Geometry: final body of the model. Coordinates: model frame, mm. Face numbers are marked on the shaded views. A direction names the side the tool comes from. Give positions to 0.01 mm unless a question says otherwise; leave off trailing zeros. Write each loop counter-clockwise with the first axis right and the second up, starting at its lowest first coordinate (ties: lowest second). Pieces come first, ordered by that corner, then holes. Notation, with made-up numbers: (68, 16) -> (98, 16) arc R21 ccw to (98, 55) -> close; hole circle Ø3 at (68, 38). An arc over 180 degrees is marked (long way). Answer as a JSON object with one key per item and string values. Group by question number.
(1) Contact query for flat-ended pins moving along their axis: pin 1 Ø2 at (x, y) = (2.5, 10) entering from +Z (3 decimals); pin 2 Ø10 at (x, z) = (4.5, 19.5) entering from +Y (3 decimals); pin 3 Ø2.5 at (x, y) = (0, 12.7) entering from +Z (1 decimal). Output: stop coordinate, or through.
(2) Set-up query: the marked faces 4 and 5. Return all of +Z, -Z, +X, -X, +Y, -Y with unobstructed straight access to the full face (end or side cutting, diameter ignored); none if empty.
(3) Draft query along Z for the marked faces 1, 2 and 3. Return one class per face: +Z half, -Z half, draft (parallel to the pull), parting line (faces both ways), or undercut.
(4) Section query A-A on y = 12.7. Output: boundary loops of the cut face in (x, z) (3 decimals).
(5) Section query B-B on z = -12.7. Output: boundary loops of the cut face in (x, y) (3 decimals), plus the area to 3 significant figures.
(6) Material intervals for probe 1 along Y at (x, z) = (0, -24.35); probe 2 along X at (y, z) = (12.7, -23.3); probe 3 along Y at (x, z) = (0, -23.5), sorted ascending.
(7) Section query C-C on x = -9. Output: boundary loops of the cut face in (y, z) (3 decimals).
(8) Section query D-D on y = 28. Output: boundary loops of the cut face in (x, z) (3 decimals).
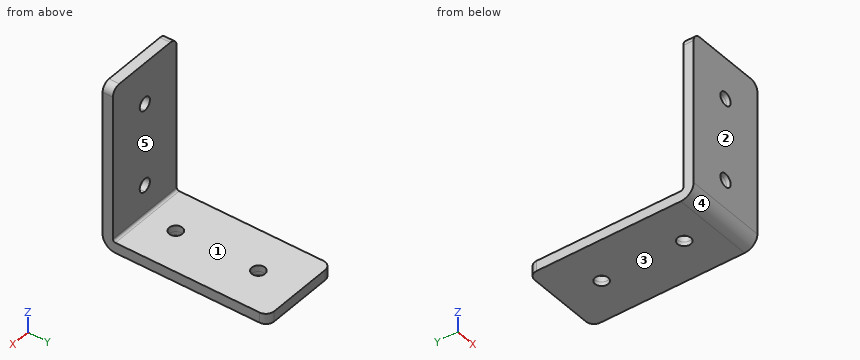
from build123d import *
from build123d.topology import SkipClean

# Parameters (mm, degrees)
SKETCH1_W                  = 25.4
SKETCH1_H                  = 50.8
SKETCH1_R                  = 2.032
BOSS_EXTRUDE1_DEPTH        = 1.27
SKETCH2_W                  = 25.4
SKETCH2_H                  = 50.8
SKETCH2_R                  = 2.032
BOSS_EXTRUDE2_DEPTH        = 1.27
CONVERT_SOLID2_START       = -24.13
CONVERT_SOLID2_OUTLINE_W   = 25.4
CONVERT_SOLID2_OUTLINE_H   = 49.53
CONVERT_SOLID2_OUTLINE_R   = 2.032
CONVERT_SOLID2_DEPTH       = 1.905
CONVERT_SOLID2_START_2     = -10.6679999
CONVERT_SOLID2_2_OUTLINE_W = 25.4
CONVERT_SOLID2_2_OUTLINE_H = 1.905
CONVERT_SOLID2_2_DEPTH     = 21.336301023
CONVERT_SOLID2_START_3     = 14.7320001
CONVERT_SOLID2_3_OUTLINE_W = 25.4
CONVERT_SOLID2_3_OUTLINE_H = 1.905
CONVERT_SOLID2_3_DEPTH     = 10.6679999
CONVERT_SOLID2_START_4     = -22.225
CONVERT_SOLID2_4_OUTLINE_W = 25.4
CONVERT_SOLID2_4_OUTLINE_H = 1.905
CONVERT_SOLID2_4_DEPTH     = 7.493301123
CONVERT_SOLID2_START_5     = 1.27
CONVERT_SOLID2_5_DEPTH     = 1.905
CONVERT_SOLID2_6_DEPTH     = 1.905
CONVERT_SOLID2_START_6     = -14
CONVERT_SOLID2_7_DEPTH     = 28
CONVERT_SOLID2_START_7     = -12.7
CONVERT_SOLID2_8_DEPTH     = 25.4
FILLET1_R                  = 2.54


with BuildPart() as part:
    # Sketch1 → Boss-Extrude1 (new body)
    with BuildSketch(Plane(origin=(0, 0, 0), x_dir=(1, 0, 0), z_dir=(0, 1, 0))):
        Rectangle(SKETCH1_W, SKETCH1_H)
        with Locations(Location((0, 12.7, 0), (0, 0, 270))):
            Circle(SKETCH1_R, mode=Mode.SUBTRACT)
        with Locations(Location((0, -12.7, 0), (0, 0, 90))):
            Circle(SKETCH1_R, mode=Mode.SUBTRACT)
    extrude(amount=BOSS_EXTRUDE1_DEPTH)

    # Sketch2 → Boss-Extrude2 (add)
    with BuildSketch(Plane(origin=(0, 0, -25.4), x_dir=(-1, 0, 0), z_dir=(0, 0, -1))):
        with Locations((0, 25.4)):
            Rectangle(SKETCH2_W, SKETCH2_H)
        with Locations((0, 12.7)):
            Circle(SKETCH2_R, mode=Mode.SUBTRACT)
        with Locations(Location((0, 38.1, 0), (0, 0, 180))):
            Circle(SKETCH2_R, mode=Mode.SUBTRACT)
    extrude(amount=-BOSS_EXTRUDE2_DEPTH)

    # Convert-Solid2: read off the stored shape, not the designer's step
    # Convert-Solid2 outline → Convert-Solid2 (add)
    with SkipClean():  # the faces are left unmerged after this step: merging them gives an invalid solid
        with BuildSketch(Plane.XY.offset(CONVERT_SOLID2_START)):
            with Locations((0, 26.035)):
                Rectangle(CONVERT_SOLID2_OUTLINE_W, CONVERT_SOLID2_OUTLINE_H)
            with Locations((0, 12.7)):
                Circle(CONVERT_SOLID2_OUTLINE_R, mode=Mode.SUBTRACT)
            with Locations((0, 38.1)):
                Circle(CONVERT_SOLID2_OUTLINE_R, mode=Mode.SUBTRACT)
        extrude(amount=CONVERT_SOLID2_DEPTH)
    add(part.part.scale(1), mode=Mode.REPLACE)  # the faces are merged on a copy

    # Convert-Solid2 2 outline → Convert-Solid2 2 (add)
    with BuildSketch(Plane.XY.offset(CONVERT_SOLID2_START_2)):
        with Locations((0, 2.2225)):
            Rectangle(CONVERT_SOLID2_2_OUTLINE_W, CONVERT_SOLID2_2_OUTLINE_H)
    extrude(amount=CONVERT_SOLID2_2_DEPTH)

    # Convert-Solid2 3 outline → Convert-Solid2 3 (add)
    with BuildSketch(Plane.XY.offset(CONVERT_SOLID2_START_3)):
        with Locations((0, 2.2225)):
            Rectangle(CONVERT_SOLID2_3_OUTLINE_W, CONVERT_SOLID2_3_OUTLINE_H)
    extrude(amount=CONVERT_SOLID2_3_DEPTH)

    # Convert-Solid2 4 outline → Convert-Solid2 4 (add)
    with BuildSketch(Plane.XY.offset(CONVERT_SOLID2_START_4)):
        with Locations((0, 2.2225)):
            Rectangle(CONVERT_SOLID2_4_OUTLINE_W, CONVERT_SOLID2_4_OUTLINE_H)
    extrude(amount=CONVERT_SOLID2_4_DEPTH)

    # Convert-Solid2 5 outline → Convert-Solid2 5 (cut)
    with BuildSketch(Plane(origin=(0, 0, 0), x_dir=(1, 0, 0), z_dir=(0, 1, 0)).offset(CONVERT_SOLID2_START_5)):
        with BuildLine():
            ThreePointArc((0.034981041, -10.668301123), (0, -10.668), (-0.034981041, -10.668301123))
            Line((-0.034981041, -10.668301123), (0.034981041, -10.668301123))
        make_face()
        with BuildLine():
            ThreePointArc((0.034981041, 14.731698877), (0, 14.732), (-0.034981041, 14.731698877))
            Line((-0.034981041, 14.731698877), (0.034981041, 14.731698877))
        make_face()
    extrude(amount=CONVERT_SOLID2_5_DEPTH, mode=Mode.SUBTRACT)

    # Convert-Solid2 6 outline → Convert-Solid2 6 (add)
    with BuildSketch(Plane(origin=(0, 0, 0), x_dir=(1, 0, 0), z_dir=(0, 1, 0)).offset(CONVERT_SOLID2_START_5)):
        with BuildLine():
            Line((-12.7, -10.668301123), (-12.7, -14.7320001))
            Line((-12.7, -14.7320001), (0, -14.732))
            ThreePointArc((0, -14.732), (-2.031924718, -12.717491168), (-0.034981041, -10.668301123))
            Line((-0.034981041, -10.668301123), (-12.7, -10.668301123))
        make_face()
        with BuildLine():
            ThreePointArc((0.034981041, -10.668301123), (2.031924718, -12.717491168), (0, -14.732))
            Line((0, -14.732), (12.7, -14.7320001))
            Line((12.7, -14.7320001), (12.7, -10.668301123))
            Line((12.7, -10.668301123), (0.034981041, -10.668301123))
        make_face()
        with BuildLine():
            Line((-12.7, 14.731698877), (-12.7, 10.6679999))
            Line((-12.7, 10.6679999), (0, 10.668))
            ThreePointArc((0, 10.668), (-2.031924718, 12.682508832), (-0.034981041, 14.731698877))
            Line((-0.034981041, 14.731698877), (-12.7, 14.731698877))
        make_face()
        with BuildLine():
            ThreePointArc((0.034981041, 14.731698877), (2.031924718, 12.682508832), (0, 10.668))
            Line((0, 10.668), (12.7, 10.6679999))
            Line((12.7, 10.6679999), (12.7, 14.731698877))
            Line((12.7, 14.731698877), (0.034981041, 14.731698877))
        make_face()
    extrude(amount=CONVERT_SOLID2_6_DEPTH)

    # Convert-Solid2 7 outline → Convert-Solid2 7 (cut)
    with SkipClean():  # the faces are left unmerged after this step: merging them gives an invalid solid
        with BuildSketch(Plane.YZ.offset(CONVERT_SOLID2_START_6)):
            with BuildLine():
                ThreePointArc((3.937, -25.4), (1.153120602, -24.246879398), (0, -21.463))
                Line((0, -21.463), (0, -25.4))
                Line((0, -25.4), (3.937, -25.4))
            make_face()
        extrude(amount=CONVERT_SOLID2_7_DEPTH, mode=Mode.SUBTRACT)

    # Convert-Solid2 8 outline → Convert-Solid2 8 (add)
    with SkipClean():  # the faces are left unmerged after this step: merging them gives an invalid solid
        with BuildSketch(Plane.YZ.offset(CONVERT_SOLID2_START_7)):
            with BuildLine():
                ThreePointArc((3.937, -22.225), (3.398184633, -22.001815367), (3.175, -21.463))
                Line((3.175, -21.463), (3.175, -22.225))
                Line((3.175, -22.225), (3.937, -22.225))
            make_face()
        extrude(amount=CONVERT_SOLID2_8_DEPTH)

    # Fillet1
    fillet1_edges = [part.edges().sort_by_distance(p)[0] for p in [
        (-12.7, 1.5875, 25.4),
        (12.7, 1.5875, 25.4),
        (12.7, 50.8, -23.8125),
        (-12.7, 50.8, -23.8125),
    ]]
    fillet(fillet1_edges, radius=FILLET1_R)


solid = part.part
Answer list:
{
 "1": {"pin 1": "z = -22.225", "pin 2": "y = 3.175", "pin 3": "through"},
 "2": {"face 4": "-Z, +X, -X, -Y", "face 5": "+Z, +X, -X, +Y"},
 "3": {"face 1": "+Z half", "face 2": "draft", "face 3": "-Z half"},
 "4": {"outline": "(-12.7, -25.4) -> (-2.032, -25.4) -> (-2.032, -22.225) -> (-12.7, -22.225) -> close; (2.032, -25.4) -> (12.7, -25.4) -> (12.7, -22.225) -> (2.032, -22.225) -> close"},
 "5": {"outline": "(-12.7, 0) -> (-2.032, 0) -> (-2.032, 3.175) -> (-12.7, 3.175) -> close; (2.032, 0) -> (12.7, 0) -> (12.7, 3.175) -> (2.032, 3.175) -> close", "area": "67.7 mm2"},
 "6": {"probe 1": "1.26 to 10.67, 14.73 to 36.07, 40.13 to 50.8", "probe 2": "-12.7 to -2.03, 2.03 to 12.7", "probe 3": "0.57 to 10.67, 14.73 to 36.07, 40.13 to 50.8"},
 "7": {"outline": "(0, -21.463) arc R3.937 ccw to (3.937, -25.4) -> (50.8, -25.4) -> (50.8, -22.225) -> (3.937, -22.225) arc R0.762 cw to (3.175, -21.463) -> (3.175, 25.4) -> (0, 25.4) -> close"},
 "8": {"outline": "(-12.7, -25.4) -> (12.7, -25.4) -> (12.7, -22.225) -> (-12.7, -22.225) -> close"}
}
